from build123d import *

# Parameters (mm, degrees)
SKETCH001_W   = 28.911368
SKETCH001_H   = 11.888076
SKETCH001_W_2 = 28.673414
SKETCH001_H_2 = 9.741194
POCKET_DEPTH  = 8.2


with BuildPart() as part:
    # Sketch → Revolution (revolve)
    with BuildSketch(Plane.XZ):
        Polygon((0, 0), (11.4, 0), (11.4, 2), (10.6, 2), (10.6, 3.5), (9, 3.5), (9, 7.7), (10.4, 8.7), (9, 11.7), (7.7, 11.7), (7.7, 3.5), (0, 3.5), align=None)
    revolve(axis=Axis((0, 0, 0), (0, 0, 1)))

    # Sketch001 (on Face9 of Revolution) → Pocket (cut)
    with BuildSketch(Plane(origin=(0, 0, 11.7), x_dir=(-1, 0, 0), z_dir=(0, 0, 1))):
        with Locations((-0.075645, 8.544038)):
            Rectangle(SKETCH001_W, SKETCH001_H)
        with Locations((0.162309, -7.470597)):
            Rectangle(SKETCH001_W_2, SKETCH001_H_2)
    extrude(amount=-POCKET_DEPTH, mode=Mode.SUBTRACT)


solid = part.part
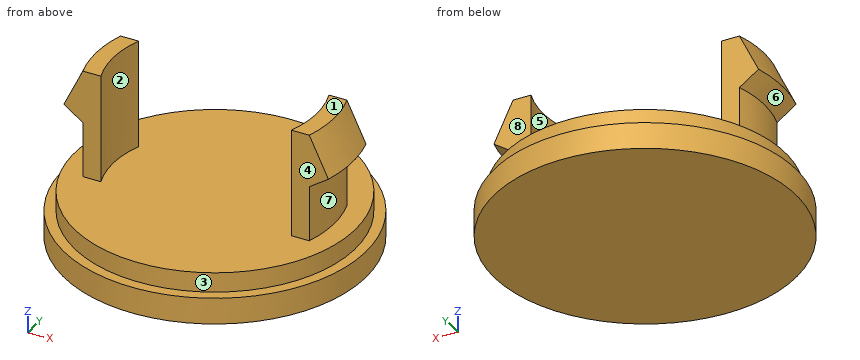
CAD build for the part. Positions are in the model's coordinates, mm. Face numbers are marked on the shaded views. A direction names the side the tool comes from. Coordinates: 2 decimals unless noted, no trailing zeros. Write each loop counter-clockwise with the first axis right and the second up, starting at its lowest first coordinate (ties: lowest second). Pieces come first, ordered by that corner, then holes. Notation, with made-up numbers: (-9, -19.5) - (-1, -19.5) arc R27 cw to (-1, 1.5) - close; hole circle Ø3 at (87, 71.25). An arc over 180 degrees is marked (long way). Use a Markdown table: item, result. Add a question column.
Item 1: 3-axis set-ups, long thin cutter, end or side, ignore diameter. For the marked faces 4, 5, 6, 7 and 8: which of +Z, -Z, +X, -X, +Y, -Y reach the whole face in a straight line?
Item 2: Flat gauge pins, fed straight in: pin 1 (11.5 mm diameter, centred on x = -1, y = 1.5, fed in from +Z); pin 2 (5 mm diameter, centred on x = -7.5, z = 4, fed in from +Y); pin 3 (0.8 mm diameter, centred on x = 8.5, z = 6.5, fed in from -Y). Where does each tip first touch, or does it go through?
Item 3: Mould opens along Y. For the marked faces 1, 2 and 3 say: pulls with the +Y half, pulls with the -Y half, needs draft (parallel to the pull), parting line crosses it, or undercut.
Item 4: Drill centre lines: L1, parallel to Z at x = 0, y = 1; L2, parallel to Y at x = 8.5, z = 10; L3, parallel to Y at x = -1.5, z = 1.75. Where is each one in solid material? Low to high. Write a range as from..to.
Item 5: Band-saw the part on B-B, the plane x = 0. Give the cut face in (y, z).
Item 6: Band-saw the part on C-C, the plane y = 0. Give the cut face in (x, z).
Item 7: Band-saw the part on D-D, the plane z = 3. Give the cut face in (x, y).
Item 8: Band-saw the part on A-A, the plane z = 6.75. Give the cut face in (x, y), and give its area (3 significant figures).
Numbers:
| question | item | result |
|---|---|---|
| 1 | face 4 | +Z, +X, -X, -Y |
| 1 | face 5 | +Z |
| 1 | face 6 | -X |
| 1 | face 7 | +X |
| 1 | face 8 | +Z, +X, -X, +Y |
| 2 | pin 1 | z = 3.5 |
| 2 | pin 2 | y = 9.69 |
| 2 | pin 3 | y = -2.6 |
| 3 | face 1 | needs draft |
| 3 | face 2 | undercut |
| 3 | face 3 | parting line crosses it |
| 4 | L1 | 0..3.5 |
| 4 | L2 | -2.6..2.6 |
| 4 | L3 | -11.3..11.3 |
| 5 | outline | (-11.4, 0) - (11.4, 0) - (11.4, 2) - (10.6, 2) - (10.6, 3.5) - (-10.6, 3.5) - (-10.6, 2) - (-11.4, 2) - close |
| 6 | outline | (-11.4, 0) - (11.4, 0) - (11.4, 2) - (10.6, 2) - (10.6, 3.5) - (9, 3.5) - (9, 7.7) - (10.4, 8.7) - (9, 11.7) - (7.7, 11.7) - (7.7, 3.5) - (-7.7, 3.5) - (-7.7, 11.7) - (-9, 11.7) - (-10.4, 8.7) - (-9, 7.7) - (-9, 3.5) - (-10.6, 3.5) - (-10.6, 2) - (-11.4, 2) - close |
| 7 | outline | circle Ø21.2 at (0, 0) |
| 8 | outline | (-8.62, -2.6) - (-7.25, -2.6) arc R7.7 cw to (-7.25, 2.6) - (-8.62, 2.6) arc R9 ccw to start; (7.25, -2.6) - (8.62, -2.6) arc R9 ccw to (8.62, 2.6) - (7.25, 2.6) arc R7.7 cw to start |
| 8 | area | 13.8 mm2 |
